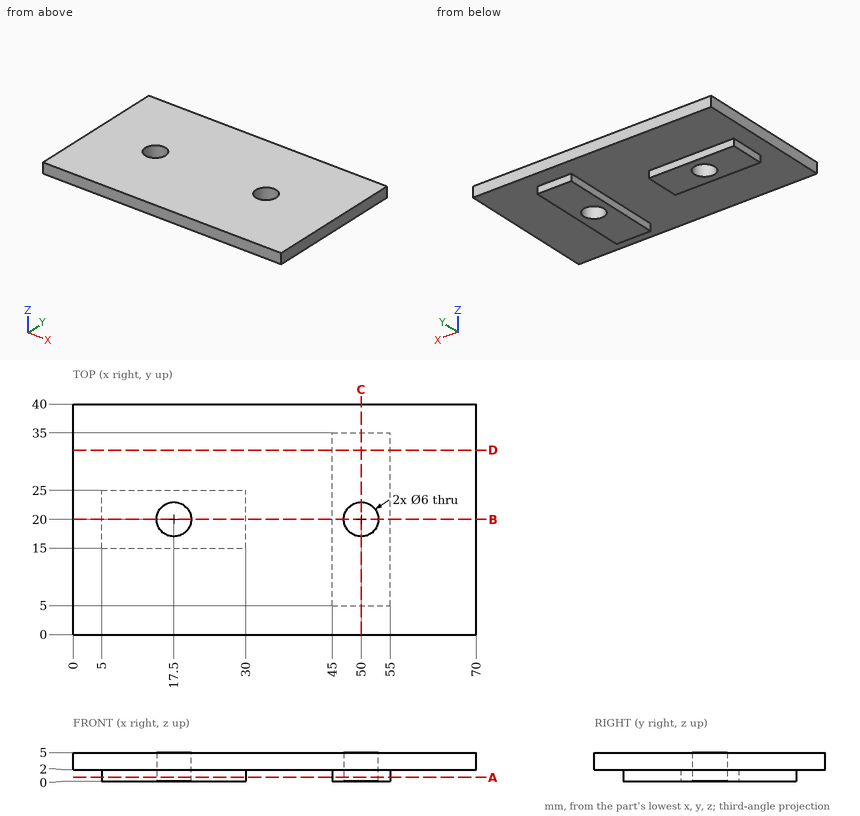
Job drawing, mm, ordinate dimensions from the low corner. One solid piece. Coordinates: 2 decimals unless noted, no trailing zeros. Order: outer loops, then holes, each group sorted by start corner. A loop starts at its lowest first (then second) coordinate and runs counter-clockwise, first axis right, second up. Notation, with made-up numbers: M 29,8 L 57,8 A32 ccw 57,45 Z; hole C 77.5,33.5 d2. An arc over 180 degrees is marked long. One line per question, with ' | ' between items.
Q1. Drill centre lines: line 1 (X direction, y = 20, z = 3.7); line 2 (X direction, y = 20, z = 1.85); line 3 (Y direction, x = 50, z = 1.3). Where is each one in solid material? Low to high.
A:
line 1: x = 0 to 14.5, 20.5 to 47, 53 to 70 | line 2: x = 5 to 14.5, 20.5 to 30, 45 to 47, 53 to 55 | line 3: y = 5 to 17, 23 to 35
Q2. Slice it at C-C (x = 50). Give the cut face in (y, z).
A:
outline: M 0,2 L 5,2 L 5,0 L 17,0 L 17,5 L 0,5 Z; M 23,0 L 35,0 L 35,2 L 40,2 L 40,5 L 23,5 Z
Q3. Slice it at B-B (y = 20). Give the cut face in (x, z).
A:
outline: M 0,2 L 5,2 L 5,0 L 14.5,0 L 14.5,5 L 0,5 Z; M 20.5,0 L 30,0 L 30,2 L 45,2 L 45,0 L 47,0 L 47,5 L 20.5,5 Z; M 53,0 L 55,0 L 55,2 L 70,2 L 70,5 L 53,5 Z
Q4. Slice it at A-A (z = 0.7). Give the cut face in (x, y).
A:
outline: M 5,15 L 30,15 L 30,25 L 5,25 Z; M 45,5 L 55,5 L 55,35 L 45,35 Z; hole C 17.5,20 d6; hole C 50,20 d6
Q5. Slice it at D-D (y = 32). Give the cut face in (x, z), and give its area (3 significant figures).
A:
outline: M 0,2 L 45,2 L 45,0 L 55,0 L 55,2 L 70,2 L 70,5 L 0,5 Z | area: 230 mm^2
Q6. Pin check, flat tips, straight feed: P1, Ø1, axis at x = 48.5, z = 1, coming from the +Y side; P2, Ø1, axis at x = 15.5, z = 1, coming from the +Y side; P3, Ø0.6, axis at y = 21.5, z = 1.5, coming from the -X side. Stop position of each tip, or through.
A:
P1: stops at y = 35 | P2: stops at y = 25 | P3: stops at x = 5
